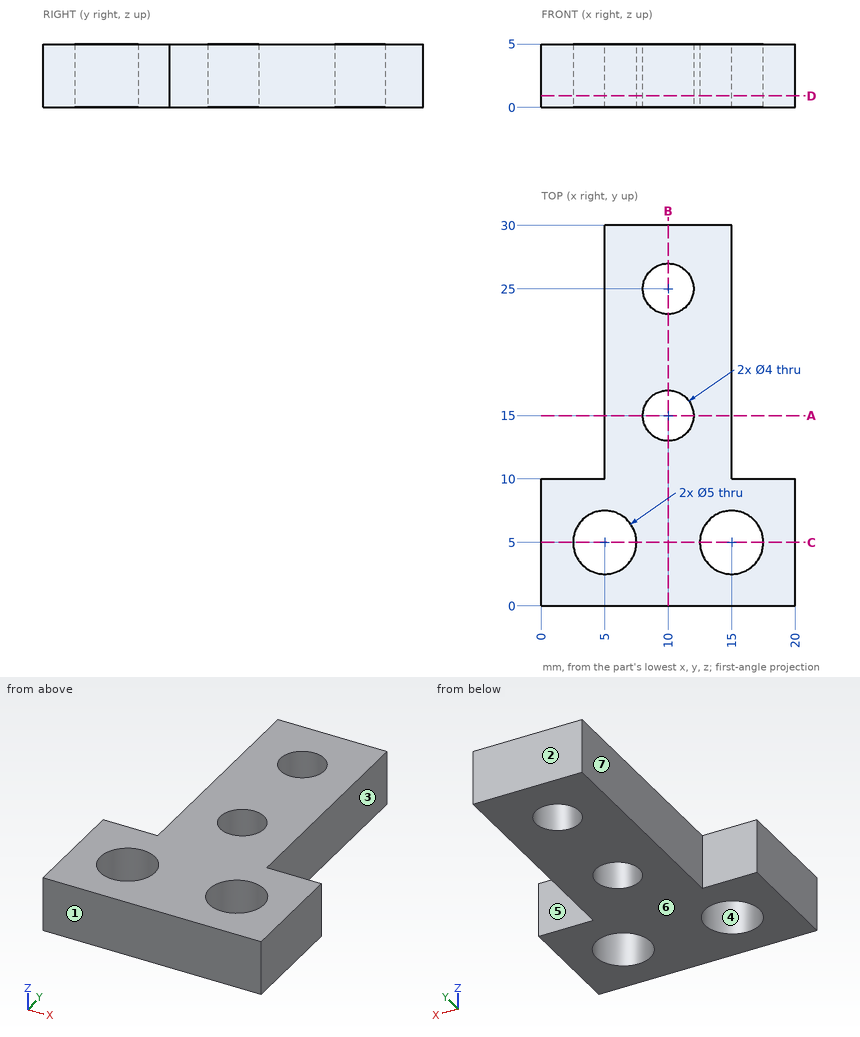
Design review of the part shown in the three views and the two pictorial views. Dimensions are in mm from the part's minimum x, y and z. A direction names the side the tool comes from. Give positions to 0.01 mm unless a question says otherwise; leave off trailing zeros. Write each loop counter-clockwise with the first axis right and the second up, starting at its lowest first coordinate (ties: lowest second). Pieces come first, ordered by that corner, then holes.
Item 1: Insertion check: P1, Ø1.5, axis at y = 19.5, z = 3, coming from the -X side; P2, Ø3, axis at x = 10, y = 25, coming from the -Z side. Each pin has a flat end and moves straight along its axis. Give the tip position at first contact, or say it passes through.
Item 2: Take a section at B-B (x = 10). Give the boundary of the cut face in (y, z).
Item 3: The part is to be moulded in two halves that separate along Y. For the marked faces 1, 2, 3 and 4, say which applies: +Y half, -Y half, draft (parallel to the pull), parting line (faces both ways), or undercut.
Item 4: Take a section at D-D (z = 0.9). Give the boundary of the cut face in (x, y).
Item 5: Take a section at A-A (y = 15). Give the boundary of the cut face in (x, z), and give its area (3 significant figures).
Item 6: Wall thickness on probe 1 along Y at (x, z) = (10, 2.6); probe 2 along X at (y, z) = (7, 0.6); probe 3 along X at (y, z) = (4.25, 3.05): over which ranges is each line inside the solid? List them lowest first.
Item 7: Take a section at C-C (y = 5). Give the boundary of the cut face in (x, z).
Item 8: Machinability: for the marked faces 5, 6 and 7, which of the approach directions +Z, -Z, +X, -X, +Y, -Y give a long, thin tool a straight path to every point of the face, cutting with its end or side? Answer none if there is none.
Established:
1. P1: stops at x = 5
1. P2: passes through
2. outline: (0, 0) - (13, 0) - (13, 5) - (0, 5) - close; (17, 0) - (23, 0) - (23, 5) - (17, 5) - close; (27, 0) - (30, 0) - (30, 5) - (27, 5) - close
3. face 1: -Y half
3. face 2: +Y half
3. face 3: draft
3. face 4: undercut
4. outline: (0, 0) - (20, 0) - (20, 10) - (15, 10) - (15, 30) - (5, 30) - (5, 10) - (0, 10) - close; hole circle Ø5 at (5, 5); hole circle Ø4 at (10, 15); hole circle Ø4 at (10, 25); hole circle Ø5 at (15, 5)
5. outline: (5, 0) - (8, 0) - (8, 5) - (5, 5) - close; (12, 0) - (15, 0) - (15, 5) - (12, 5) - close
5. area: 30.0 mm2
6. probe 1: y = 0 to 13, 17 to 23, 27 to 30
6. probe 2: x = 0 to 3.5, 6.5 to 13.5, 16.5 to 20
6. probe 3: x = 0 to 2.62, 7.38 to 12.62, 17.38 to 20
7. outline: (0, 0) - (2.5, 0) - (2.5, 5) - (0, 5) - close; (7.5, 0) - (12.5, 0) - (12.5, 5) - (7.5, 5) - close; (17.5, 0) - (20, 0) - (20, 5) - (17.5, 5) - close
8. face 5: +Z, -Z, +X, +Y
8. face 6: -Z, +X, -X, +Y, -Y
8. face 7: +Z, -Z, -X, +Y
